For this review, take the finished solid that the model builds, in its own axes (mm). Face numbers are marked on the shaded views. A direction names the side the tool comes from. Coordinates: 2 decimals unless noted, no trailing zeros. Loops run counter-clockwise (first coordinate to the right, second up) from the corner with the lowest first, then second, coordinate; pieces in that order, holes last. Notation, with made-up numbers: (72.25, -3) - (109.25, -3) arc R27 ccw to (109.25, 18) - close; hole circle Ø2 at (58, 29.5). An arc over 180 degrees is marked (long way). Answer as a JSON object with one key per item and string values. Group by question number.
Item 1: Tool access review of the marked faces 1 and 2: name each direction out of +Z, -Z, +X, -X, +Y, -Y from which nothing blocks a thin tool from reaching the whole face with its end or side.
Item 2: We need section B-B (x = 470). Give the boundary of the cut face in (y, z), then the cut area to 3 significant figures.
Item 3: Clearance check with flat-ended pins moving along their axes: pin 1 (1 mm diameter, centred on x = 489, z = -60.5, fed in from -Y); pin 2 (4 mm diameter, centred on x = 451, z = 63.5, fed in from +Y); pin 3 (7.5 mm diameter, centred on x = 455, z = -59, fed in from -Y); pin 4 (1.6 mm diameter, centred on x = 489.5, y = -142, fed in from +Z). State where each tip first meets the part, or that it passes through.
Item 4: We need section C-C (y = -91.5). Give the boundary of the cut face in (x, z), then the cut area to 3 significant figures.
Item 5: We need section A-A (y = -43.5). Give the boundary of the cut face in (x, z).
Item 6: To check wall thickness, follow line 1 (Y direction, x = 489, z = 47); line 2 (Y direction, x = 489, z = -8); line 3 (Z direction, x = 451, y = -0.8). State the ranges of each line that lie inside material, in increasing order.
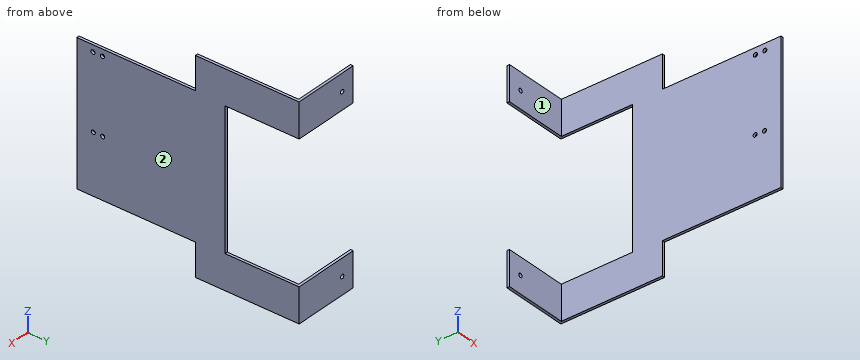
from build123d import *

# Parameters (mm, degrees)
SKETCH2_W             = 49
SKETCH2_H             = 25.5
SKETCH2_R             = 1.5
BOSS_EXTRUDE1_DEPTH   = 2
BOSS_EXTRUDE1_2_DEPTH = 2
SKETCH3_W             = 2
SKETCH3_H             = 25.5
BOSS_EXTRUDE2_DEPTH   = 53
SKETCH4_W             = 152.5
SKETCH4_H             = 22
SKETCH4_W_2           = 104
SKETCH4_H_2           = 88
SKETCH4_R             = 1.5
BOSS_EXTRUDE3_DEPTH   = 2


with BuildPart() as part:
    # Sketch2 → Boss-Extrude1 (new body)
    with BuildSketch(Plane.XZ):
        with Locations((465.5, -63.5)):
            Rectangle(SKETCH2_W, SKETCH2_H)
        with Locations((451, -63.5)):
            Circle(SKETCH2_R, mode=Mode.SUBTRACT)
    extrude(amount=BOSS_EXTRUDE1_DEPTH)



with BuildPart() as body_2:
    # Sketch2 → Boss-Extrude1 2 (new body)
    with BuildSketch(Plane.XZ):
        with Locations((465.5, 63.5)):
            Rectangle(SKETCH2_W, SKETCH2_H)
        with Locations((451, 63.5)):
            Circle(SKETCH2_R, mode=Mode.SUBTRACT)
    extrude(amount=BOSS_EXTRUDE1_2_DEPTH)


with BuildPart() as part_1:
    add(part.part)

    add(body_2.part)  # Boss-Extrude2 merges body 2
    # Sketch3 → Boss-Extrude2 (add)
    with BuildSketch(Plane.XZ.offset(2)):
        with Locations((489, 63.5)):
            Rectangle(SKETCH3_W, SKETCH3_H)
        with Locations((489, -63.5)):
            Rectangle(SKETCH3_W, SKETCH3_H)
    extrude(amount=BOSS_EXTRUDE2_DEPTH)

    # Sketch4 → Boss-Extrude3 (add)
    with BuildSketch(Plane(origin=(490, 0, 0), x_dir=(0, 0, -1), z_dir=(1, 0, 0))):
        with Locations((0, -66)):
            Rectangle(SKETCH4_W, SKETCH4_H)
        with Locations((0, -121)):
            Rectangle(SKETCH4_W_2, SKETCH4_H_2)
        with Locations((-47, -146)):
            Circle(SKETCH4_R, mode=Mode.SUBTRACT)
        with Locations((-47, -153)):
            Circle(SKETCH4_R, mode=Mode.SUBTRACT)
        with Locations((7.999524512, -145.771300426)):
            Circle(SKETCH4_R, mode=Mode.SUBTRACT)
        with Locations((8, -152.77130041)):
            Circle(SKETCH4_R, mode=Mode.SUBTRACT)
    extrude(amount=-BOSS_EXTRUDE3_DEPTH)


solid = part_1.part
Check sheet entries:
{
 "1": {"face 1": "+Z, -Z, -X, -Y", "face 2": "+Z, -Z, +X, +Y, -Y"},
 "2": {"outline": "(-2, -76.25) - (0, -76.25) - (0, -50.75) - (-2, -50.75) - close; (-2, 50.75) - (0, 50.75) - (0, 76.25) - (-2, 76.25) - close", "area": "102 mm2"},
 "3": {"pin 1": "stops at y = -77", "pin 2": "stops at y = 0", "pin 3": "stops at y = -2", "pin 4": "stops at z = 52"},
 "4": {"outline": "(488, -52) - (490, -52) - (490, 52) - (488, 52) - close", "area": "208 mm2"},
 "5": {"outline": "(488, -76.25) - (490, -76.25) - (490, -50.75) - (488, -50.75) - close; (488, 50.75) - (490, 50.75) - (490, 76.25) - (488, 76.25) - close"},
 "6": {"line 1": "y = -165 to -154.5, -151.5 to -147.5, -144.5 to -55", "line 2": "y = -165 to -154.27, -151.27 to -147.27, -144.27 to -55", "line 3": "z = -76.25 to -65, -62 to -50.75, 50.75 to 62, 65 to 76.25"}
}
